The listing builds one solid part. Answer for the finished solid, in the listing's coordinates (mm). A direction names the side the tool comes from. Give positions to 0.01 mm unless a question says otherwise; leave off trailing zeros. Write each loop counter-clockwise with the first axis right and the second up, starting at its lowest first coordinate (ties: lowest second). Pieces come first, ordered by that corner, then holes. Notation, with made-up numbers: (19, -6.5) -> (74, -6.5) arc R4 ccw to (74, 0.5) -> close; hole circle Ø5 at (62, 75). An arc over 180 degrees is marked (long way). One line per question, with ' | ' between items.
from build123d import *

# Parameters (mm, degrees)
F0_W     = 203.2
F0_H     = 127
F1_DEPTH = 127
F3_DEPTH = 76.2
F4_SIZE2 = 101.6
F4_SIZE  = 76.2
F5_R     = 5.08


# Not quite as in the source:
# - the program builds the solid bodies; features that only make, move or delete a surface that nothing else refers to are left out


with BuildPart() as f1:
    # F0 (on Front) → F1 (new body)
    with BuildSketch(Plane.XZ):
        Rectangle(F0_W, F0_H)
    extrude(amount=F1_DEPTH)

    # F2 (on face) → F3 (cut)
    with BuildSketch(Plane.XZ.offset(127)):
        Polygon((-40.63635692, -6.0839741491), (-40.63635692, -63.5), (101.6, -63.5), (101.6, 63.5), (7.1171009913, 63.5), (7.1171009913, -6.0839741491), align=None)
    extrude(amount=-F3_DEPTH, mode=Mode.SUBTRACT)

    # F4
    f4_edges = [f1.edges().sort_by_distance(p)[0] for p in [
        (101.6, -25.4, 63.5),
    ]]
    f4_side = f1.faces().sort_by_distance((-21.033148, -53.671887, 63.5))[0]
    chamfer(f4_edges, length=F4_SIZE, length2=F4_SIZE2, reference=f4_side)

    # F5
    f5_edges = [f1.edges().sort_by_distance(p)[0] for p in [
        (-47.24145, -127, 63.5),
        (7.117101, -127, 28.708013),
        (7.117101, -88.9, -6.083974),
        (7.117101, -88.9, 63.5),
        (16.25855, -50.8, 63.5),
        (25.4, -25.4, 63.5),
        (-16.759628, -127, -6.083974),
        (-40.636357, -127, -34.791987),
        (-71.118178, -127, -63.5),
        (-101.6, -127, 0),
        (-101.6, -63.5, 63.5),
        (-101.6, -63.5, -63.5),
        (-101.6, 0, 0),
        (-38.1, 0, 63.5),
        (0, 0, -63.5),
    ]]
    fillet(f5_edges, radius=F5_R)


solid = f1.part
Item 1: Find section A-A (y = -67). Write down the section's boundary in (x, z).
Answers below:
outline: (-101.6, -58.42) arc R5.08 ccw to (-96.52, -63.5) -> (-40.64, -63.5) -> (-40.64, -6.08) -> (2.04, -6.08) arc R5.08 ccw to (7.12, -1) -> (7.12, 58.42) arc R5.08 ccw to (2.04, 63.5) -> (-96.52, 63.5) arc R5.08 ccw to (-101.6, 58.42) -> close
Item 2: Find section C-C (x = -16.5). Write down the section's boundary in (y, z).
Answers below:
outline: (-127, -1) arc R5.08 ccw to (-121.92, -6.08) -> (-50.8, -6.08) -> (-50.8, -63.5) -> (-5.08, -63.5) arc R5.08 ccw to (0, -58.42) -> (0, 58.42) arc R5.08 ccw to (-5.08, 63.5) -> (-121.92, 63.5) arc R5.08 ccw to (-127, 58.42) -> close
Item 3: Flat-ended cylindrical pins translate along their axes: pin 1 (2 mm diameter, centred on y = -22.5, z = 5, fed in from +X) (3 decimals); pin 2 (3 mm diameter, centred on x = -37.5, y = -79.5, fed in from -Z); pin 3 (6 mm diameter, centred on y = -113.5, z = 41, fed in from +X). Find the tip coordinate at first contact, or state that the pin passes through.
Answers below:
pin 1: x = 70.025 | pin 2: z = -6.08 | pin 3: x = 7.12
Item 4: Find section B-B (z = 13.5). Write down the section's boundary in (x, y).
Answers below:
outline: (-101.6, -121.92) arc R5.08 ccw to (-96.52, -127) -> (2.04, -127) arc R5.08 ccw to (7.12, -121.92) -> (7.12, -50.8) -> (62.9, -50.8) -> (62.9, 0) -> (-96.52, 0) arc R5.08 ccw to (-101.6, -5.08) -> close
Item 5: Consider line 1 (X direction, y = -73, z = 19); line 2 (Y direction, x = 25, z = -44); line 3 (X direction, y = -114, z = -9.5). Determine where each line is inside the solid, lowest interval first. Write a range as [from, to].
Answers below:
line 1: [-101.6, 7.12] | line 2: [-50.8, 0] | line 3: [-101.6, -40.64]
Item 6: A tool of negligible diameter and unlimited length cuts with its end or side. For faces 1 (the face through (5.668, -85.862, -4.556)), 2 (the face through (-101.6, -63, -1)), 3 (the face through (15.433, -49.272, 62.051)), from which of +Z, -Z, +X, -X, +Y, -Y can it reach the whole face along a straight path? Write none if from no direction.
Answers below:
face 1: -Z, +X, -Y | face 2: +Z, -Z, -X, +Y, -Y | face 3: +Z, +X, -Y
Item 7: Find section D-D (y = -23). Write down the section's boundary in (x, z).
Answers below:
outline: (-101.6, -58.42) arc R5.08 ccw to (-96.52, -63.5) -> (101.6, -63.5) -> (101.6, -38.1) -> (26.92, 61.47) arc R5.08 ccw to (22.86, 63.5) -> (-96.52, 63.5) arc R5.08 ccw to (-101.6, 58.42) -> close
